```python
from build123d import *

# Parameters (mm, degrees)
BOSS_EXTRUDE1_DEPTH = 3
CUT_EXTRUDE1_REACH  = 42.606
SKETCH2_R           = 2.5
CUT_EXTRUDE2_REACH  = 42.606


with BuildPart() as part:
    # Sketch1 → Boss-Extrude1 (new body)
    with BuildSketch(Plane(origin=(0, 0, 0), x_dir=(0, 1, 0), z_dir=(0, 0, 1))):
        with BuildLine():
            Line((-16.529411765, 4.794117647), (36.210588235, 4.794117647))
            ThreePointArc((36.210588235, 4.794117647), (40.210588235, 0.794117647), (36.210588235, -3.205882353))
            Line((36.210588235, -3.205882353), (-16.529411765, -3.205882353))
            ThreePointArc((-16.529411765, -3.205882353), (-20.529411765, 0.794117647), (-16.529411765, 4.794117647))
        make_face()
    extrude(amount=BOSS_EXTRUDE1_DEPTH)

    # Sketch2 → Cut-Extrude1 (cut, up to next)
    with BuildSketch(Plane.XY.offset(3), mode=Mode.PRIVATE) as cut_extrude1_sk1:
        with Locations((-0.794117647, -16.529411765)):
            Circle(SKETCH2_R)
    cut_extrude1_tool1 = extrude(cut_extrude1_sk1.sketch, amount=-CUT_EXTRUDE1_REACH, mode=Mode.PRIVATE) & part.part
    # Sketch2 → Cut-Extrude1 (cut, up to next)
    with BuildSketch(Plane.XY.offset(3), mode=Mode.PRIVATE) as cut_extrude1_sk2:
        with Locations((-0.794117647, 36.210588235)):
            Circle(SKETCH2_R)
    cut_extrude1_tool2 = extrude(cut_extrude1_sk2.sketch, amount=-CUT_EXTRUDE1_REACH, mode=Mode.PRIVATE) & part.part
    add(cut_extrude1_tool1.solids().sort_by_distance((-0.794118, -16.529412, 3))[0], mode=Mode.SUBTRACT)
    add(cut_extrude1_tool2.solids().sort_by_distance((-0.794118, 36.210588, 3))[0], mode=Mode.SUBTRACT)

    # Sketch3 → Cut-Extrude2 (cut, up to next)
    with BuildSketch(Plane.XY.offset(3), mode=Mode.PRIVATE) as cut_extrude2_sk1:
        with BuildLine():
            Line((-2.645474442, -6.529411765), (-2.645474442, 26.210588235))
            ThreePointArc((-2.645474442, 26.210588235), (-0.645474442, 28.210588235), (1.354525558, 26.210588235))
            Line((1.354525558, 26.210588235), (1.354525558, -6.529411765))
            ThreePointArc((1.354525558, -6.529411765), (-0.645474442, -8.529411765), (-2.645474442, -6.529411765))
        make_face()
    cut_extrude2_tool1 = extrude(cut_extrude2_sk1.sketch, amount=-CUT_EXTRUDE2_REACH, mode=Mode.PRIVATE) & part.part
    add(cut_extrude2_tool1.solids().sort_by_distance((-0.645474, 9.840588, 3))[0], mode=Mode.SUBTRACT)


solid = part.part
```
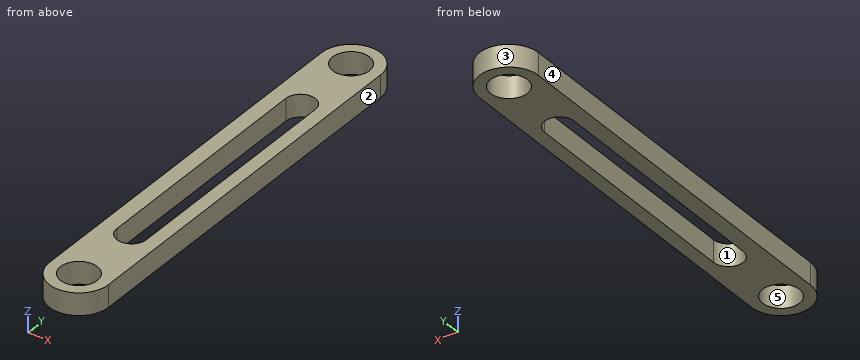
Model file for the job. Use its own axes, mm. Face numbers are marked on the shaded views. A direction names the side the tool comes from. Coordinates: 2 decimals unless noted, no trailing zeros. Loops run counter-clockwise (first coordinate to the right, second up) from the corner with the lowest first, then second, coordinate; pieces in that order, holes last. Notation, with made-up numbers: (17, 58.5) - (52, 58.5) arc R15 cw to (52, 70.5) - close; hole circle Ø3 at (-32.5, 31). An arc over 180 degrees is marked (long way). Answer as a JSON object with one key per item and string values. Group by question number.
(1) Tool access for the marked faces 1 and 2: list every direction of +Z, -Z, +X, -X, +Y, -Y with a clear straight run to the whole face (end or side of a thin tool).
(2) Probe line 1 along Y through (x, z) = (-0.75, 2.5); line 2 along X through (y, z) = (-5.5, 2.8); line 3 along Y through (x, z) = (-3, 2.85). List the from-to ranges inside material, lowest first.
(3) Two-plate mould, pull along Y, no slides. Class the marked faces 3, 4 and 5: released by +Y, released by -Y, zero draft, split by the parting line, or undercut.
(4) Flat gauge pin, fed straight in: pin 1 (1 mm diameter, centred on x = 0.5, z = 1.5, fed in from -Y). Where does the tip first touch, or does it go through?
(5) Cut at A-A (z = 2.3). Give the cut face in (x, y).
(6) Cut at D-D (x = -4). Give the cut face in (y, z), then the cut area to 3 significant figures.
(7) Cut at C-C (x = 0). Give the cut face in (y, z).
(8) Cut at B-B (y = 35). Give the cut face in (x, z), then the cut area to 3 significant figures.
Geometry says:
{
 "1": {"face 1": "+Z, -Z", "face 2": "+Z, -Z, +X, +Y, -Y"},
 "2": {"line 1": "y = -20.53 to -19.03, -14.03 to -8.53, 28.21 to 33.71, 38.71 to 40.21", "line 2": "x = -4.79 to -2.65, 1.35 to 3.21", "line 3": "y = -19.87 to -17.71, -15.35 to 35.03, 37.39 to 39.55"},
 "3": {"face 3": "released by +Y", "face 4": "zero draft", "face 5": "undercut"},
 "4": {"pin 1": "stops at y = -20.45"},
 "5": {"outline": "(-4.79, -16.53) arc R4 ccw to (3.21, -16.53) - (3.21, 36.21) arc R4 ccw to (-4.79, 36.21) - close; hole circle Ø5 at (-0.79, -16.53); hole circle Ø5 at (-0.79, 36.21); hole (-2.65, -6.53) arc R2 ccw to (1.35, -6.53) - (1.35, 26.21) arc R2 ccw to (-2.65, 26.21) - close"},
 "6": {"outline": "(-18.92, 0) - (38.6, 0) - (38.6, 3) - (-18.92, 3) - close", "area": "173 mm^2"},
 "7": {"outline": "(-20.45, 0) - (-18.9, 0) - (-18.9, 3) - (-20.45, 3) - close; (-14.16, 0) - (-8.42, 0) - (-8.42, 3) - (-14.16, 3) - close; (28.1, 0) - (33.84, 0) - (33.84, 3) - (28.1, 3) - close; (38.58, 0) - (40.13, 0) - (40.13, 3) - (38.58, 3) - close"},
 "8": {"outline": "(-4.79, 0) - (-2.98, 0) - (-2.98, 3) - (-4.79, 3) - close; (1.39, 0) - (3.21, 0) - (3.21, 3) - (1.39, 3) - close", "area": "10.9 mm^2"}
}
